from build123d import *

# Parameters (mm, degrees)
SKETCH1_W                  = 33.528
SKETCH1_H                  = 33.02
BOSS_EXTRUDE1_DEPTH        = 3.175
CUT_EXTRUDE1_DEPTH         = 4.175
SKETCH3_W                  = 3.29438
SKETCH3_H                  = 8.37692
BOSS_EXTRUDE2_DEPTH        = 3.175
CUT_EXTRUDE2_DEPTH         = 7.35
SKETCH5_W                  = 3.29438
SKETCH5_H                  = 8.37692
BOSS_EXTRUDE3_DEPTH        = 3.175
CUT_EXTRUDE3_DEPTH         = 7.35
SKETCH7_W                  = 3.29438
SKETCH7_H                  = 8.37692
BOSS_EXTRUDE4_DEPTH        = 3.175
CUT_EXTRUDE4_DEPTH         = 7.35
SKETCH9_W                  = 3.29438
SKETCH9_H                  = 8.37692
BOSS_EXTRUDE5_DEPTH        = 3.175
CUT_EXTRUDE5_DEPTH         = 3.175
CUT_EXTRUDE6_DEPTH         = 3.175
CUT_EXTRUDE7_DEPTH         = 3.175
CUT_EXTRUDE8_DEPTH         = 3.175
HOLE1_D                    = 12.7254
HOLE1_DEPTH                = 3.175025
M2_5_CLEARANCE_HOLE1_D     = 2.7051
M2_5_CLEARANCE_HOLE1_DEPTH = 3.175025
M3_CLEARANCE_HOLE1_D       = 3.556
M3_CLEARANCE_HOLE1_DEPTH   = 3.175025
M2_5_CLEARANCE_HOLE2_D     = 2.7051
M2_5_CLEARANCE_HOLE2_DEPTH = 3.29438
M2_5_CLEARANCE_HOLE3_D     = 2.7051
M2_5_CLEARANCE_HOLE3_DEPTH = 3.29438
M2_5_CLEARANCE_HOLE4_D     = 2.7051
M2_5_CLEARANCE_HOLE4_DEPTH = 3.29443
FILLET1_R                  = 0.635
FILLET2_R                  = 3.175


with BuildPart() as part:
    # Sketch1 → Boss-Extrude1 (new body)
    with BuildSketch(Plane.XZ):
        Rectangle(SKETCH1_W, SKETCH1_H)
    extrude(amount=-BOSS_EXTRUDE1_DEPTH)

    # Sketch2 → Cut-Extrude1 (cut, through all)
    with BuildSketch(Plane(origin=(0, 3.175, 0), x_dir=(-1, 0, 0), z_dir=(0, 1, 0))):
        with BuildLine():
            Line((-13.46962, 16.51), (-13.46962, 10.753335779))
            ThreePointArc((-13.46962, 10.753335779), (-11.652039651, 8.508623021), (-8.8307675, 9.127296717))
            ThreePointArc((-8.8307675, 9.127296717), (0, 12.7), (8.8307675, 9.127296717))
            ThreePointArc((8.8307675, 9.127296717), (11.652039651, 8.508623021), (13.46962, 10.753335779))
            Line((13.46962, 10.753335779), (13.46962, 16.51))
            Line((13.46962, 16.51), (-13.46962, 16.51))
        make_face()
    extrude(amount=-CUT_EXTRUDE1_DEPTH, mode=Mode.SUBTRACT)

    # Sketch3 → Boss-Extrude2 (add)
    with BuildSketch(Plane.XZ):
        with Locations((-15.11681, 12.32154)):
            Rectangle(SKETCH3_W, SKETCH3_H)
    extrude(amount=BOSS_EXTRUDE2_DEPTH)

    # Sketch4 → Cut-Extrude2 (cut, through all)
    with BuildSketch(Plane(origin=(0, 3.175, 0), x_dir=(-1, 0, 0), z_dir=(0, 1, 0))):
        with BuildLine():
            Line((-16.764, 8.13308), (-16.764, -8.13308))
            Line((-16.764, -8.13308), (-12.593680427, -1.639882101))
            ThreePointArc((-12.593680427, -1.639882101), (-12.7, 0), (-12.593680427, 1.639882101))
            Line((-12.593680427, 1.639882101), (-16.764, 8.13308))
        make_face()
    extrude(amount=-CUT_EXTRUDE2_DEPTH, mode=Mode.SUBTRACT)

    # Sketch5 → Boss-Extrude3 (add)
    with BuildSketch(Plane.XZ):
        with Locations((15.11681, 12.32154)):
            Rectangle(SKETCH5_W, SKETCH5_H)
    extrude(amount=BOSS_EXTRUDE3_DEPTH)

    # Sketch6 → Cut-Extrude3 (cut, through all)
    with BuildSketch(Plane(origin=(0, 3.175, 0), x_dir=(-1, 0, 0), z_dir=(0, 1, 0))):
        with BuildLine():
            Line((13.46962, -16.51), (13.46962, -10.753335779))
            ThreePointArc((13.46962, -10.753335779), (11.652039651, -8.508623021), (8.8307675, -9.127296717))
            ThreePointArc((8.8307675, -9.127296717), (0, -12.7), (-8.8307675, -9.127296717))
            ThreePointArc((-8.8307675, -9.127296717), (-11.652039651, -8.508623021), (-13.46962, -10.753335779))
            Line((-13.46962, -10.753335779), (-13.46962, -16.51))
            Line((-13.46962, -16.51), (13.46962, -16.51))
        make_face()
    extrude(amount=-CUT_EXTRUDE3_DEPTH, mode=Mode.SUBTRACT)

    # Sketch7 → Boss-Extrude4 (add)
    with BuildSketch(Plane.XZ):
        with Locations((15.11681, -12.32154)):
            Rectangle(SKETCH7_W, SKETCH7_H)
    extrude(amount=BOSS_EXTRUDE4_DEPTH)

    # Sketch8 → Cut-Extrude4 (cut, through all)
    with BuildSketch(Plane(origin=(0, 3.175, 0), x_dir=(-1, 0, 0), z_dir=(0, 1, 0))):
        with BuildLine():
            Line((16.764, -8.13308), (16.764, 8.13308))
            Line((16.764, 8.13308), (12.593680427, 1.639882101))
            ThreePointArc((12.593680427, 1.639882101), (12.7, 0), (12.593680427, -1.639882101))
            Line((12.593680427, -1.639882101), (16.764, -8.13308))
        make_face()
    extrude(amount=-CUT_EXTRUDE4_DEPTH, mode=Mode.SUBTRACT)

    # Sketch9 → Boss-Extrude5 (add)
    with BuildSketch(Plane.XZ):
        with Locations((-15.11681, -12.32154)):
            Rectangle(SKETCH9_W, SKETCH9_H)
    extrude(amount=BOSS_EXTRUDE5_DEPTH)

    # Sketch10 → Cut-Extrude5 (cut)
    with BuildSketch(Plane.XZ.offset(3.175)):
        with BuildLine():
            Line((15.422429016, -8.13308), (13.46962, -8.13308))
            Line((13.46962, -8.13308), (13.46962, -10.329337463))
            ThreePointArc((13.46962, -10.329337463), (14.503938678, -9.282703292), (15.422429016, -8.13308))
        make_face()
    extrude(amount=-CUT_EXTRUDE5_DEPTH, mode=Mode.SUBTRACT)

    # Sketch11 → Cut-Extrude6 (cut)
    with BuildSketch(Plane.XZ.offset(3.175)):
        with BuildLine():
            Line((13.46962, 10.329337463), (13.46962, 8.13308))
            Line((13.46962, 8.13308), (15.422429016, 8.13308))
            ThreePointArc((15.422429016, 8.13308), (14.503938678, 9.282703292), (13.46962, 10.329337463))
        make_face()
    extrude(amount=-CUT_EXTRUDE6_DEPTH, mode=Mode.SUBTRACT)

    # Sketch12 → Cut-Extrude7 (cut)
    with BuildSketch(Plane.XZ.offset(3.175)):
        with BuildLine():
            Line((-15.422429016, 8.13308), (-13.46962, 8.13308))
            Line((-13.46962, 8.13308), (-13.46962, 10.329337463))
            ThreePointArc((-13.46962, 10.329337463), (-14.503938678, 9.282703292), (-15.422429016, 8.13308))
        make_face()
    extrude(amount=-CUT_EXTRUDE7_DEPTH, mode=Mode.SUBTRACT)

    # Sketch13 → Cut-Extrude8 (cut)
    with BuildSketch(Plane.XZ.offset(3.175)):
        with BuildLine():
            Line((-13.46962, -10.329337463), (-13.46962, -8.13308))
            Line((-13.46962, -8.13308), (-15.422429016, -8.13308))
            ThreePointArc((-15.422429016, -8.13308), (-14.503938678, -9.282703292), (-13.46962, -10.329337463))
        make_face()
    extrude(amount=-CUT_EXTRUDE8_DEPTH, mode=Mode.SUBTRACT)

    # Hole1
    with Locations(Plane(origin=(0, 0, 0), x_dir=(-1, 0, 0), z_dir=(0, -1, 0))):
        with Locations((0, 0)):
            Hole(HOLE1_D / 2, depth=HOLE1_DEPTH)

    # M2.5 Clearance Hole1
    with Locations(Plane(origin=(0, 0, 0), x_dir=(-1, 0, 0), z_dir=(0, -1, 0))):
        with Locations((0, -9.779), (9.779, 0), (0, 9.779), (-9.779, 0)):
            Hole(M2_5_CLEARANCE_HOLE1_D / 2, depth=M2_5_CLEARANCE_HOLE1_DEPTH)

    # M3 Clearance Hole1
    with Locations(Plane(origin=(0, 0, 0), x_dir=(-1, 0, 0), z_dir=(0, -1, 0))):
        with Locations((6.914797213, -6.914797213), (6.914797213, 6.914797213), (-6.914797213, 6.914797213), (-6.914797213, -6.914797213)):
            Hole(M3_CLEARANCE_HOLE1_D / 2, depth=M3_CLEARANCE_HOLE1_DEPTH)

    # M2.5 Clearance Hole2
    with Locations(Plane(origin=(16.764, 0, 0), x_dir=(0, 0, -1), z_dir=(1, 0, 0))):
        with Locations((13.470384182, 0)):
            Hole(M2_5_CLEARANCE_HOLE2_D / 2, depth=M2_5_CLEARANCE_HOLE2_DEPTH)

    # M2.5 Clearance Hole3
    with Locations(Plane.ZY.offset(-13.46962)):
        with Locations((13.470384182, 0)):
            Hole(M2_5_CLEARANCE_HOLE3_D / 2, depth=M2_5_CLEARANCE_HOLE3_DEPTH)

    # M2.5 Clearance Hole4
    with Locations(Plane(origin=(-13.46962, 0, 0), x_dir=(0, 0, -1), z_dir=(1, 0, 0))):
        with Locations((-13.470384182, 0), (13.470384182, 0)):
            Hole(M2_5_CLEARANCE_HOLE4_D / 2, depth=M2_5_CLEARANCE_HOLE4_DEPTH)

    # Fillet1
    fillet1_edges = [part.edges().sort_by_distance(p)[0] for p in [
        (-13.46962, -1.5875, -10.329337463),
        (-15.422429016, -1.5875, 8.13308),
        (15.422429016, -1.5875, -8.13308),
        (15.422429016, -1.5875, 8.13308),
        (13.46962, -1.5875, -10.329337463),
        (-13.46962, -1.5875, 10.329337463),
        (-15.422429016, -1.5875, -8.13308),
        (13.46962, -1.5875, 10.329337463),
    ]]
    fillet(fillet1_edges, radius=FILLET1_R)

    # Fillet2
    fillet2_edges = [part.edges().sort_by_distance(p)[0] for p in [
        (-12.593680427, 1.5875, -1.639882101),
        (12.593680427, 1.5875, -1.639882101),
        (-12.593680427, 1.5875, 1.639882101),
        (12.593680427, 1.5875, 1.639882101),
    ]]
    fillet(fillet2_edges, radius=FILLET2_R)


solid = part.part
Part model, mm, in its own coordinate system. A direction names the side the tool comes from. Give positions to 0.01 mm unless a question says otherwise; leave off trailing zeros. Order: outer loops, then holes, each group sorted by start corner. A loop starts at its lowest first (then second) coordinate and runs counter-clockwise, first axis right, second up. Notation, with made-up numbers: (52, 22) - (81, 22) arc R30 ccw to (81, 56) - close; hole circle Ø2 at (-28, 57). An arc over 180 degrees is marked (long way). One line per question, with ' | ' between items.
1. Band-saw the part on C-C on z = -4.5. List the corners of the cut face in (x, y) (3 decimals), then the cut area to 3 significant figures.
Filled in:
outline: (-14.431, 0) - (-4.498, 0) - (-4.498, 3.175) - (-14.431, 3.175) - close; (4.498, 0) - (14.431, 0) - (14.431, 3.175) - (4.498, 3.175) - close | area: 63.1 mm²
2. Band-saw the part on B-B on x = 0. List the corners of the cut face in (y, z) (3 decimals), then the cut area to 3 significant figures.
Filled in:
outline: (0, -12.7) - (3.175, -12.7) - (3.175, -11.132) - (0, -11.132) - close; (0, -8.426) - (3.175, -8.426) - (3.175, -6.363) - (0, -6.363) - close; (0, 6.363) - (3.175, 6.363) - (3.175, 8.426) - (0, 8.426) - close; (0, 11.132) - (3.175, 11.132) - (3.175, 12.7) - (0, 12.7) - close | area: 23.1 mm²
3. Pull direction X, two halves, no side cores. Call faces 1 (the face through (-16.764, 0, -11)), 2 (the face through (16.764, 0, -11)), 3 (the face through (15, -3.175, 12)), 4 (the face through (14.5, -1.61, 9.29)): +X half, -X half, draft (parallel to the pull), parting line (faces both ways), or undercut.
Filled in:
face 1: -X half | face 2: +X half | face 3: draft | face 4: undercut
4. Which spindle directions (+Z, -Z, +X, -X, +Y, -Y) get a long thin tool onto all of the face, cutting with end or side? Do faces 5 (the face through (-13.47, 0, 15)), 6 (the face through (-0.29, 1.61, 11.1)), 7 (the face through (14.948, 1.61, 5.305)). Say none if no direction does.
Filled in:
face 5: +Z, +Y, -Y | face 6: +Y, -Y | face 7: +X, +Y, -Y
5. Band-saw the part on D-D on z = 0. List the corners of the cut face in (x, y) (3 decimals).
Filled in:
outline: (-12.7, 0) - (-11.132, 0) - (-11.132, 3.175) - (-12.7, 3.175) - close; (-8.426, 0) - (-6.363, 0) - (-6.363, 3.175) - (-8.426, 3.175) - close; (6.363, 0) - (8.426, 0) - (8.426, 3.175) - (6.363, 3.175) - close; (11.132, 0) - (12.7, 0) - (12.7, 3.175) - (11.132, 3.175) - close
6. Band-saw the part on A-A on y = -2.5. List the corners of the cut face in (x, z) (3 decimals).
Filled in:
outline: (-16.764, -16.51) - (-13.47, -16.51) - (-13.47, -10.606) arc R0.635 ccw to (-13.668, -10.145) arc R13.97 cw to (-15.236, -8.387) arc R0.635 ccw to (-15.744, -8.133) - (-16.764, -8.133) - close; (-16.764, 8.133) - (-15.744, 8.133) arc R0.635 ccw to (-15.236, 8.387) arc R13.97 cw to (-13.668, 10.145) arc R0.635 ccw to (-13.47, 10.606) - (-13.47, 16.51) - (-16.764, 16.51) - close; (13.47, -16.51) - (16.764, -16.51) - (16.764, -8.133) - (15.744, -8.133) arc R0.635 ccw to (15.236, -8.387) arc R13.97 cw to (13.668, -10.145) arc R0.635 ccw to (13.47, -10.606) - close; (13.47, 10.606) arc R0.635 ccw to (13.668, 10.145) arc R13.97 cw to (15.236, 8.387) arc R0.635 ccw to (15.744, 8.133) - (16.764, 8.133) - (16.764, 16.51) - (13.47, 16.51) - close
7. Drill centre lines: probe 1 along Z at (x, y) = (-5.5, 1.25); probe 2 along Z at (x, y) = (0, 1.2); probe 3 along X at (y, z) = (1.25, -10.5). Where is each one in solid material? Low to high.
Filled in:
probe 1: -11.45 to -7.99, -5.84 to -3.2, 3.2 to 5.84, 7.99 to 11.45 | probe 2: -12.7 to -11.13, -8.43 to -6.36, 6.36 to 8.43, 11.13 to 12.7 | probe 3: -16.76 to -13.42, -7.14 to -1.14, 1.14 to 7.14, 13.42 to 16.76
8. Drop flat-ended pins along their axis: P1, Ø3, axis at x = 6.91, z = -6.91, coming from the +Y side; P2, Ø3, axis at x = 10.5, z = 0, coming from the -Y side; P3, Ø1.5, axis at x = -7.5, y = -0.5, coming from the -Z side. Give the stop position or say it passes through.
Filled in:
P1: through | P2: y = 0 | P3: z = -10.64
